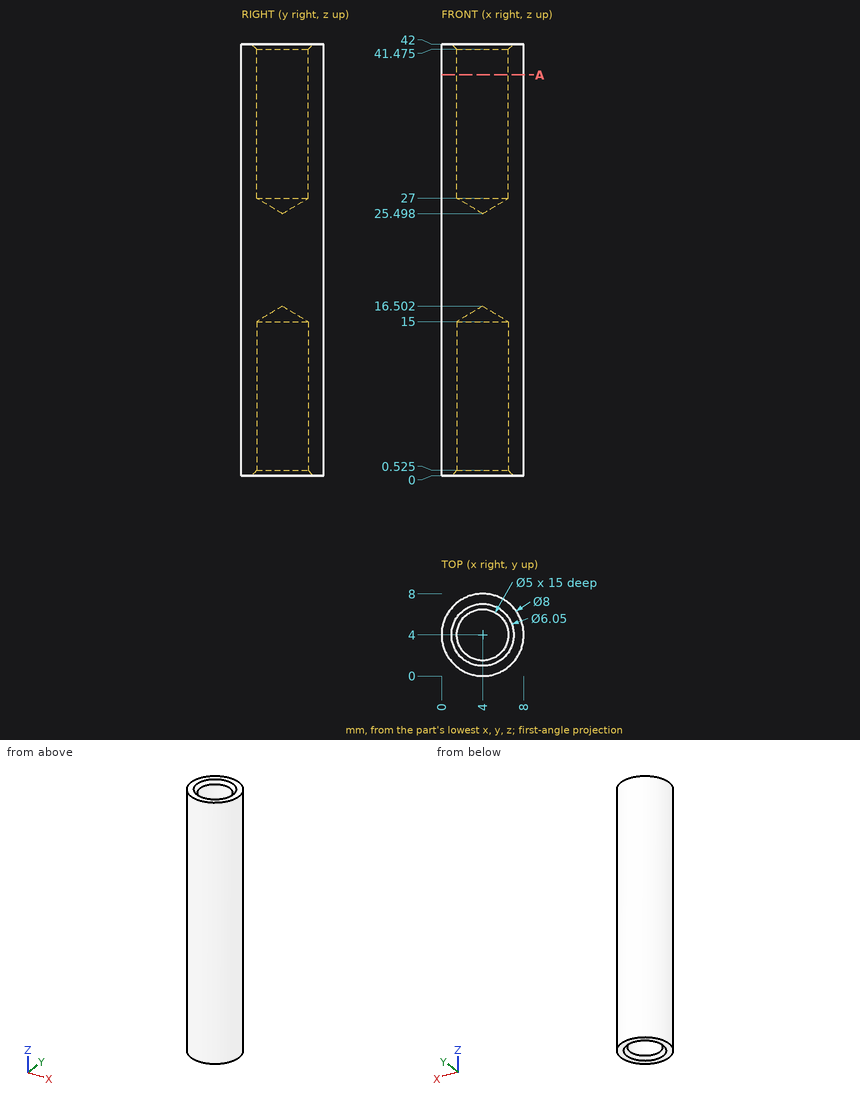
Part print with two shaded views. Sizes in mm from the minimum x, y, z corner. Round coordinates to 2 decimals unless told otherwise and drop trailing zeros. Loops run counter-clockwise (first coordinate to the right, second up) from the corner with the lowest first, then second, coordinate; pieces in that order, holes last. Notation, with made-up numbers: M -11.75,83.5 L 24.25,83.5 A21 ccw 24.25,109.5 Z; hole C -22,57 d9. An arc over 180 degrees is marked long. Return JSON: item names as keys, results as strings. Group by question number.
(1) Drop flat-ended pins along their axis: P1, Ø1.5, axis at x = 3, z = 33.5, coming from the -Y side; P2, Ø1.5, axis at x = 6, z = 7.5, coming from the -Y side; P3, Ø4.5, axis at x = 4, y = 4, coming from the -Z side; P4, Ø1, axis at x = 2.5, y = 1.5, coming from the -Z side. Give the stop position or say it passes through.
(2) Saw through at A-A, the plane z = 39. List the corners of the cut face in (x, y), and give its area (3 significant figures).
(3) Wall check: probe 1 along Y at (x, z) = (4, 10.5); probe 2 along X at (y, z) = (3.25, 8) (1 decimal); probe 3 along Y at (x, z) = (3.5, 3.5). Give the ranges that are in metal, low to high. Write a range as [from, to].
Answer list:
{
 "1": {"P1": "y = 0.01", "P2": "y = 0.2", "P3": "z = 15.15", "P4": "z = 0"},
 "2": {"outline": "C 4,4 d8; hole C 4,4 d5", "area": "30.6 mm2"},
 "3": {"probe 1": "[0, 1.5], [6.5, 8]", "probe 2": "[0.1, 1.6], [6.4, 7.9]", "probe 3": "[0.03, 1.55], [6.45, 7.97]"}
}
